Work out the finished part from the listing and answer in its coordinate system (mm). A direction names the side the tool comes from. Coordinates: 2 decimals unless noted, no trailing zeros. Order: outer loops, then holes, each group sorted by start corner. A loop starts at its lowest first (then second) coordinate and runs counter-clockwise, first axis right, second up. Notation, with made-up numbers: (39, -12.75) -> (63, -12.75) arc R21 ccw to (63, 25.25) -> close; hole circle Ø10 at (58, -19). An arc over 180 degrees is marked (long way). Answer as CSV lines item,"result". Start each with the question number.
Item 1: Section C-C (x = -70) is taken. Write down the section's boundary in (y, z).
Item 2: Which of the six approach directions +Z, -Z, +X, -X, +Y, -Y give full straight-line access (tool end or side, diameter ignored) to faces 4 (the face through (120, -49, 3)), 5 (the face through (-90, -25, 3)), 6 (the face through (70, -20, 3))?
Item 3: Section B-B (z = 11) is taken. Write down the section's boundary in (x, y).
Item 4: For a pull along Y with two mould halves and no side action, classify faces 1 (the face through (90, -25, 3)), 2 (the face through (70, -80, 3)), 3 (the face through (-2, -49, -9.722)) as pulls with the +Y half, pulls with the -Y half, needs draft (parallel to the pull), parting line crosses it, or undercut.
Item 5: Section A-A (y = -32) is taken. Write down the section's boundary in (x, z).
Item 6: Straight lines are drawn through the part: L1, parallel to X at y = -63, z = 1.5; L2, parallel to Z at x = -90, y = -14.25; L3, parallel to X at y = -21, z = 1. For each, find the intervals that lie inside material, in ascending order.
Item 7: This flat-tipped pin is pushed along its axis until it touches: pin 1 Ø5 at (x, z) = (90.5, 1) entering from +Y. Where does it stop, or does it pass through?
Item 8: Section D-D (y = -17.5) is taken. Write down the section's boundary in (x, z).
```python
from build123d import *

# Parameters (mm, degrees)
CROQUIS1_W              = 240
CROQUIS1_H              = 25
SALIENTE_EXTRUIR1_DEPTH = 100
CROQUIS3_R              = 5
CORTAR_EXTRUIR1_DEPTH   = 25
CORTAR_EXTRUIR2_DEPTH   = 25


with BuildPart() as part:
    # Croquis1 → Saliente-Extruir1 (new body)
    with BuildSketch(Plane(origin=(0, 0, 0), x_dir=(1, 0, 0), z_dir=(0, 1, 0))):
        with Locations((0, -2.777777778)):
            Rectangle(CROQUIS1_W, CROQUIS1_H)
    extrude(amount=-SALIENTE_EXTRUIR1_DEPTH)

    # Croquis3 → Cortar-Extruir1 (cut)
    with BuildSketch(Plane(origin=(0, 0, 0), x_dir=(1, 0, 0), z_dir=(0, 1, 0))):
        with Locations((-90, -2.777777778)):
            Circle(CROQUIS3_R)
        with Locations((90, -2.777777778)):
            Circle(CROQUIS3_R)
    extrude(amount=-CORTAR_EXTRUIR1_DEPTH, mode=Mode.SUBTRACT)

    # Croquis4 → Cortar-Extruir2 (cut)
    with BuildSketch(Plane.XY.offset(15.277777778)):
        with BuildLine():
            Line((-75, -25), (-75, -75))
            ThreePointArc((-75, -75), (-70, -80), (-65, -75))
            Line((-65, -75), (-65, -25))
            ThreePointArc((-65, -25), (-70, -20), (-75, -25))
        make_face()
        with BuildLine():
            Line((65, -25), (65, -75))
            ThreePointArc((65, -75), (70, -80), (75, -75))
            Line((75, -75), (75, -25))
            ThreePointArc((75, -25), (70, -20), (65, -25))
        make_face()
    extrude(amount=-CORTAR_EXTRUIR2_DEPTH, mode=Mode.SUBTRACT)


solid = part.part
```
Checked values:
1,outline,"(-100, -9.72) -> (-80, -9.72) -> (-80, 15.28) -> (-100, 15.28) -> close; (-20, -9.72) -> (0, -9.72) -> (0, 15.28) -> (-20, 15.28) -> close"
2,face 4,"+Z, -Z, +X, +Y, -Y"
2,face 5,"+Y"
2,face 6,"+Z, -Z"
3,outline,"(-120, -100) -> (120, -100) -> (120, 0) -> (-120, 0) -> close; hole (-75, -75) arc R5 ccw to (-65, -75) -> (-65, -25) arc R5 ccw to (-75, -25) -> close; hole (65, -75) arc R5 ccw to (75, -75) -> (75, -25) arc R5 ccw to (65, -25) -> close"
4,face 1,"pulls with the +Y half"
4,face 2,"undercut"
4,face 3,"needs draft"
5,outline,"(-120, -9.72) -> (-75, -9.72) -> (-75, 15.28) -> (-120, 15.28) -> close; (-65, -9.72) -> (65, -9.72) -> (65, 15.28) -> (-65, 15.28) -> close; (75, -9.72) -> (120, -9.72) -> (120, 15.28) -> (75, 15.28) -> close"
6,L1,"x = -120 to -75, -65 to 65, 75 to 120"
6,L2,"z = -9.72 to -2.22, 7.78 to 15.28"
6,L3,"x = -120 to -94.67, -85.33 to -73, -67 to 67, 73 to 85.33, 94.67 to 120"
7,pin 1,"stops at y = -25"
8,outline,"(-120, -9.72) -> (120, -9.72) -> (120, 15.28) -> (-120, 15.28) -> close; hole circle Ø10 at (-90, 2.78); hole circle Ø10 at (90, 2.78)"
